For this review, take the finished solid that the model builds, in its own axes (mm). Coordinates: 2 decimals unless noted, no trailing zeros. Loops run counter-clockwise (first coordinate to the right, second up) from the corner with the lowest first, then second, coordinate; pieces in that order, holes last. Notation, with made-up numbers: (43, -17.5) - (79, -17.5) arc R18 ccw to (79, 16.5) - close; hole circle Ø10 at (79, -24.75). An arc over 180 degrees is marked (long way). One line per item, written item: value. Start each with the question number.
1. Take a section at B-B, the plane z = 0.2. State the section outline as (x, y) points, and give its area (3 significant figures).
2. Insertion check: pin 1 (1.5 mm diameter, centred on x = -16, z = 0.5, fed in from +Y). The pin has a flat end and moves straight along its axis. Give the tip position at first contact, or say it passes through.
3. Take a section at A-A, the plane x = 14. State the section outline as (y, z) points.
4. To check wall thickness, follow line 1 (Y direction, x = 15.5, z = 0.85); line 2 (Y direction, x = 15, z = -1.1); line 3 (Z direction, x = -5, y = 8.25). State the ranges of each line that lie inside material, in increasing order. Write a range as from..to.
```python
from build123d import *

# Parameters (mm, degrees)
F1_DEPTH = 1.75
F3_DEPTH = 100


with BuildPart() as f1:
    # F0 (on Top) → F1 (new body, symmetric)
    with BuildSketch(Plane.XY):
        with BuildLine():
            Line((-29.05, -12.5), (29.05, -12.5))
            ThreePointArc((29.05, -12.5), (29.757107, -12.207107), (30.05, -11.5))
            Line((30.05, -11.5), (30.05, 12.5))
            Line((30.05, 12.5), (-30.05, 12.5))
            Line((-30.05, 12.5), (-30.05, -11.5))
            ThreePointArc((-30.05, -11.5), (-29.757107, -12.207107), (-29.05, -12.5))
        make_face()
    extrude(amount=F1_DEPTH, both=True)

    # F2 (on face) → F3 (cut)
    with BuildSketch(Plane.YZ.offset(30.05)):
        Polygon((12.5, -0.75), (11.5, -1.75), (13.169873, -1.75), (13.169873, 1.75), (8.169873, 1.75), align=None)
    extrude(amount=-F3_DEPTH, mode=Mode.SUBTRACT)


solid = f1.part
```
Solutions:
1. outline: (-30.05, -11.5) arc R1 ccw to (-29.05, -12.5) - (29.05, -12.5) arc R1 ccw to (30.05, -11.5) - (30.05, 10.85) - (-30.05, 10.85) - close
1. area: 1,400 mm2
2. pin 1: y = 11.63
3. outline: (-12.5, -1.75) - (11.5, -1.75) - (12.5, -0.75) - (8.17, 1.75) - (-12.5, 1.75) - close
4. line 1: -12.5..9.73
4. line 2: -12.5..12.15
4. line 3: -1.75..1.7
